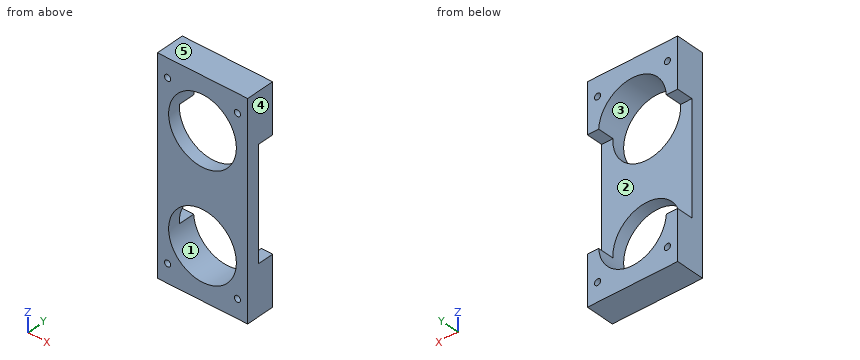
from build123d import *

# Parameters (mm, degrees)
SKETCH_1_W             = 22
SKETCH_1_H             = 51
EXTRUDE_410_DEPTH      = 3
SKETCH_2_W             = 22
SKETCH_2_H             = 12
EXTRUDE_754_DEPTH      = 4
SKETCH_3_R             = 8.25
CUT_EXTRUDE_970_DEPTH  = 8
SKETCH_4_R             = 0.75
CUT_EXTRUDE_1248_DEPTH = 8


with BuildPart() as part:
    # 草图1 → Extrude 410 (new body)
    with BuildSketch(Plane(origin=(0, 0, 0), x_dir=(1, 0, 0), z_dir=(0, 1, 0))):
        Rectangle(SKETCH_1_W, SKETCH_1_H)
    extrude(amount=EXTRUDE_410_DEPTH)

    # 草图2 → Extrude 754 (add)
    with BuildSketch(Plane(origin=(0, 3, 0), x_dir=(1, 0, 0), z_dir=(0, 1, 0))):
        with Locations((0, -19.5)):
            Rectangle(SKETCH_2_W, SKETCH_2_H)
        with Locations((0, 19.5)):
            Rectangle(SKETCH_2_W, SKETCH_2_H)
    extrude(amount=EXTRUDE_754_DEPTH)

    # 草图3 → Cut-Extrude 970 (cut, through all)
    with BuildSketch(Plane.XZ):
        with Locations((0, 13)):
            Circle(SKETCH_3_R)
        with Locations((0, -13)):
            Circle(SKETCH_3_R)
    extrude(amount=-CUT_EXTRUDE_970_DEPTH, mode=Mode.SUBTRACT)

    # 草图4 → Cut-Extrude 1248 (cut, through all)
    with BuildSketch(Plane(origin=(0, 7, 0), x_dir=(1, 0, 0), z_dir=(0, 1, 0))):
        with Locations((-8.5, -21)):
            Circle(SKETCH_4_R)
        with Locations((8.5, -21)):
            Circle(SKETCH_4_R)
        with Locations((8.5, 21)):
            Circle(SKETCH_4_R)
        with Locations((-8.5, 21)):
            Circle(SKETCH_4_R)
    extrude(amount=-CUT_EXTRUDE_1248_DEPTH, mode=Mode.SUBTRACT)


solid = part.part
Geometry: final body of the model. Coordinates: model frame, mm. Face numbers are marked on the shaded views. A direction names the side the tool comes from. Round coordinates to 2 decimals unless told otherwise and drop trailing zeros. Loops run counter-clockwise (first coordinate to the right, second up) from the corner with the lowest first, then second, coordinate; pieces in that order, holes last. Notation, with made-up numbers: (76.5, 62.5) -> (119.5, 62.5) arc R26 ccw to (119.5, 86.5) -> close; hole circle Ø6 at (-18.75, -35.75). An arc over 180 degrees is marked (long way). One line per question, with ' | ' between items. Start each with the question number.
1. Section A-A on x = 0. Output: boundary loops of the cut face in (y, z), and give its area (3 significant figures).
2. Set-up query: the marked faces 1 and 2. Return all of +Z, -Z, +X, -X, +Y, -Y with unobstructed straight access to the full face (end or side cutting, diameter ignored); none if empty.
3. Contact query for flat-ended pins moving along their axis: pin 1 (13 mm diameter, centred on x = 0, z = -13, fed in from +Y); pin 2 (1.7 mm diameter, centred on x = 8.5, z = -21, fed in from -Y); pin 3 (11 mm diameter, centred on x = 3.5, z = -1, fed in from +Y). Output: stop coordinate, or through.
4. Section D-D on x = 4.25. Output: boundary loops of the cut face in (y, z), and give its area (3 significant figures).
5. Section B-B on y = 2.5. Output: boundary loops of the cut face in (x, z).
6. Section C-C on z = -13. Output: boundary loops of the cut face in (x, y), and give its area (3 significant figures).
7. Mould query, pull axis Z, two halves, no side actions, for the marked faces 3, 4 and 5. Classes: pulls with the +Z half, pulls with the -Z half, needs draft (parallel to the pull), parting line crosses it, or undercut.
8. Line query: line 1 along Z through (x, y) = (-8.5, 2.75); line 2 along Z through (x, y) = (0, 4.5); line 3 along Z through (x, y) = (-4, 2.5). Output: solid intervals per line, ascending. Write a range as [from, to].
Returned:
1) outline: (0, -25.5) -> (7, -25.5) -> (7, -21.25) -> (0, -21.25) -> close; (0, -4.75) -> (3, -4.75) -> (3, 4.75) -> (0, 4.75) -> close; (0, 21.25) -> (7, 21.25) -> (7, 25.5) -> (0, 25.5) -> close | area: 88.0 mm2
2) face 1: +Y, -Y | face 2: +X, -X, +Y
3) pin 1: passes through | pin 2: stops at y = 0 | pin 3: stops at y = 3
4) outline: (0, -25.5) -> (7, -25.5) -> (7, -20.07) -> (0, -20.07) -> close; (0, -5.93) -> (3, -5.93) -> (3, 5.93) -> (0, 5.93) -> close; (0, 20.07) -> (7, 20.07) -> (7, 25.5) -> (0, 25.5) -> close | area: 112 mm2
5) outline: (-11, -25.5) -> (11, -25.5) -> (11, 25.5) -> (-11, 25.5) -> close; hole circle Ø1.5 at (-8.5, -21); hole circle Ø1.5 at (-8.5, 21); hole circle Ø16.5 at (0, -13); hole circle Ø16.5 at (0, 13); hole circle Ø1.5 at (8.5, -21); hole circle Ø1.5 at (8.5, 21)
6) outline: (-11, 0) -> (-8.25, 0) -> (-8.25, 3) -> (-11, 3) -> close; (8.25, 0) -> (11, 0) -> (11, 3) -> (8.25, 3) -> close | area: 16.5 mm2
7) face 3: undercut | face 4: needs draft | face 5: pulls with the +Z half
8) line 1: z = [-25.5, -21.75], [-20.25, 20.25], [21.75, 25.5] | line 2: z = [-25.5, -21.25], [21.25, 25.5] | line 3: z = [-25.5, -20.22], [-5.78, 5.78], [20.22, 25.5]
